Design review of the part built by this model. Coordinates are the model's own, in mm. A direction names the side the tool comes from. Coordinates: 2 decimals unless noted, no trailing zeros. Write each loop counter-clockwise with the first axis right and the second up, starting at its lowest first coordinate (ties: lowest second). Pieces come first, ordered by that corner, then holes. Notation, with made-up numbers: M 89.5,-23.75 L 130.5,-23.75 A24 ccw 130.5,-4.75 Z; hole C 19,-29 d5. An arc over 180 degrees is marked long. Write item = value, one per line.
```python
from build123d import *

# Parameters (mm, degrees)
F0_W     = 552.45
F0_H     = 279.4
F1_DEPTH = 19.05
F2_T     = -2.54
F3_R     = 2.5796875
F4_DEPTH = 2.54
F5_R     = 3.175
F6_DEPTH = 38.101


with BuildPart() as f1:
    # F0 (on Top) → F1 (new body, symmetric)
    with BuildSketch(Plane.XY):
        Rectangle(F0_W, F0_H)
    extrude(amount=F1_DEPTH, both=True)

    # F2
    f2_openings = [f1.faces().sort_by_distance(p)[0] for p in [
        (0, -139.7, 0),
        (-276.225, 0, 0),
        (0, 0, -19.05),
        (276.225, 0, 0),
    ]]
    offset(amount=F2_T, openings=f2_openings)

    # F3 (on face) → F4 (cut, through all)
    with BuildSketch(Plane(origin=(0, 139.7, 0), x_dir=(-1, 0, 0), z_dir=(0, 1, 0))):
        with Locations((-247.65, -6.35)):
            Circle(F3_R)
        with Locations((0, -6.35)):
            Circle(F3_R)
        with Locations((247.65, -6.35)):
            Circle(F3_R)
    extrude(amount=-F4_DEPTH, mode=Mode.SUBTRACT)

    # F5 (on face) → F6 (cut, through all)
    with BuildSketch(Plane.XY.offset(19.05)):
        with Locations((-247.65, -127)):
            Circle(F5_R)
        with Locations((0, -127)):
            Circle(F5_R)
        with Locations((247.65, -127)):
            Circle(F5_R)
    extrude(amount=-F6_DEPTH, mode=Mode.SUBTRACT)


solid = f1.part
```
Q1. Consider section A-A, the plane y = -69.5. State the section outline as (x, z) points (3 decimals).
Check result:
outline = M -276.225,16.51 L 276.225,16.51 L 276.225,19.05 L -276.225,19.05 Z
Q2. For P1, Ø4.5, axis at x = 247.65, z = -6.35, coming from the +Y side; P2, Ø1, axis at x = -89, y = 20.5, coming from the -Z side; P3, Ø6, axis at x = -247.65, z = -6.35, coming from the -Y side, all flat-tipped, find the tip position at first contact; note any pin that passes through.
Check result:
P1 = through
P2 = 16.51
P3 = 137.16
Q3. Consider section B-B, the plane z = 2. State the section outline as (x, y) points (3 decimals).
Check result:
outline = M -276.225,137.16 L 276.225,137.16 L 276.225,139.7 L -276.225,139.7 Z
Q4. Consider section C-C, the plane x = 202. State the section outline as (y, z) points.
Check result:
outline = M -139.7,16.51 L 137.16,16.51 L 137.16,-19.05 L 139.7,-19.05 L 139.7,19.05 L -139.7,19.05 Z
Q5. Wall thickness on line 1 (Y direction, x = 247.65, z = 17.1) (3 decimals); line 2 (Z direction, x = -247, y = 138); line 3 (Y direction, x = 247, z = 17): over which ranges is each line inside the solid? List them lowest first.
Check result:
line_1 = -139.7 to -130.175, -123.825 to 139.7
line_2 = -19.05 to -8.85, -3.85 to 19.05
line_3 = -139.7 to -130.11, -123.89 to 139.7
Q6. Machinability: for faces 1 (the flat face through (-4, 2, 19.05)), 2 (the flat face through (-4, 1, 16.51)), which of the approach directions +Z, -Z, +X, -X, +Y, -Y give a long, thin tool a straight path to every point of the face, cutting with its end or side? Answer none if there is none.
Check result:
face_1 = +Z, +X, -X, +Y, -Y
face_2 = -Z, +X, -X, -Y
